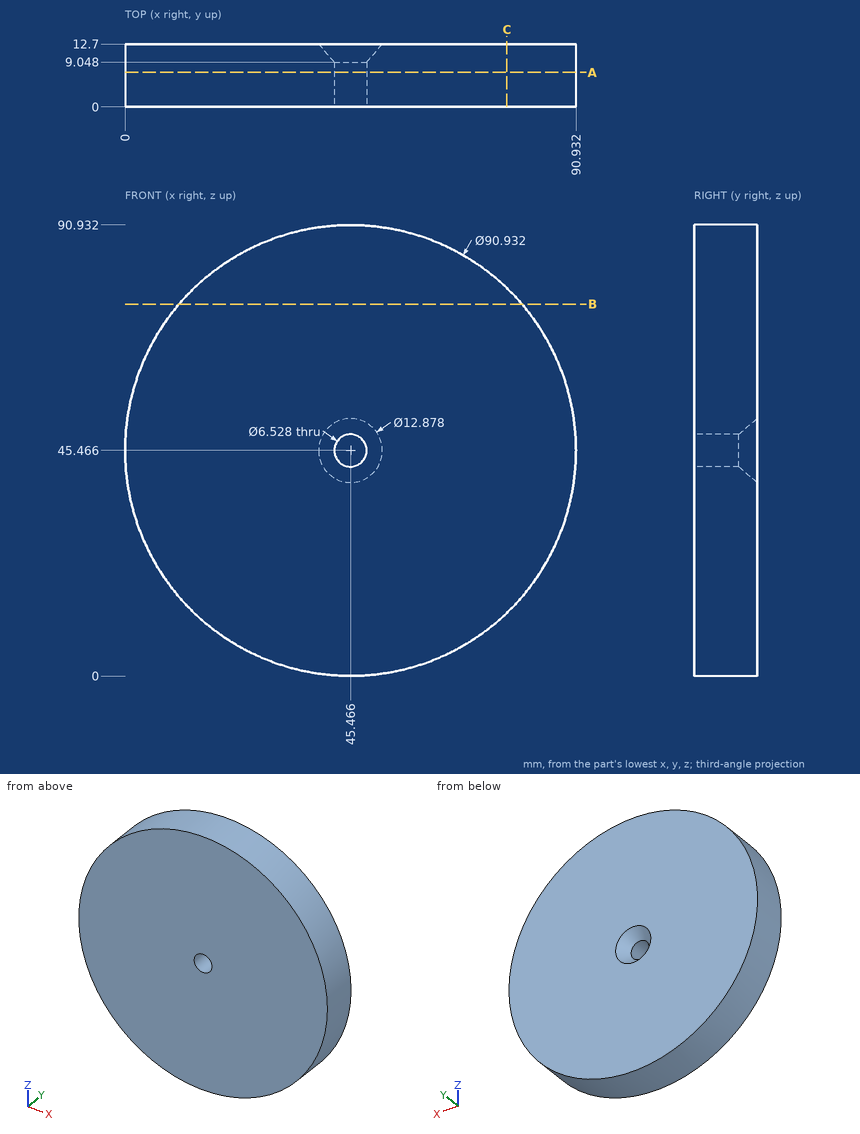
The drawing under review shows one solid part. Ordinate dimensions are in mm from its lowest x, y, z. Give positions to 0.01 mm unless a question says otherwise; leave off trailing zeros. Write each loop counter-clockwise with the first axis right and the second up, starting at its lowest first coordinate (ties: lowest second). Pieces come first, ordered by that corner, then holes. Notation, with made-up numbers: (-23.5, -20.5) -> (-18.5, -20.5) arc R12 ccw to (-18.5, -4.5) -> close; hole circle Ø3 at (35.25, 75). An arc over 180 degrees is marked (long way). Answer in a Markdown table with one row per item.
(1) Clearance check with flat-ended pins moving along their axes: pin 1 (3 mm diameter, centred on x = 58.5, y = 2.5, fed in from +Z) (1 decimal); pin 2 (1.5 mm diameter, centred on x = 24, y = 2.5, fed in from +Z); pin 3 (1.5 mm diameter, centred on y = 2.5, z = 21, fed in from +X). State where each tip first meets the part, or that it passes through.
Results:
| item | result |
|---|---|
| pin 1 | z = 89.4 |
| pin 2 | z = 85.94 |
| pin 3 | x = 84.26 |
(2) To check wall thickness, follow probe 1 along Z at (x, y) = (47, 6.5) (1 decimal); probe 2 along Y at (x, z) = (40.5, 46). State the ranges of each line that lie inside material, in increasing order.
Results:
| item | result |
|---|---|
| probe 1 | 0 to 42.6, 48.3 to 90.9 |
| probe 2 | 0 to 11.04 |
(3) Consider section B-B (z = 75). State the section outline as (x, y) points, then the cut area to 3 significant figures.
Results:
| item | result |
|---|---|
| outline | (10.9, 0) -> (80.03, 0) -> (80.03, 12.7) -> (10.9, 12.7) -> close |
| area | 878 mm2 |
(4) Consider section A-A (y = 7). State the section outline as (x, z) points, then the cut area to 3 significant figures.
Results:
| item | result |
|---|---|
| outline | circle Ø90.93 at (45.47, 45.47); hole circle Ø6.53 at (45.47, 45.47) |
| area | 6,460 mm2 |
(5) Consider section C-C (x = 77). State the section outline as (y, z) points.
Results:
| item | result |
|---|---|
| outline | (0, 12.71) -> (12.7, 12.71) -> (12.7, 78.22) -> (0, 78.22) -> close |
